Source: three-view drawing plus pictorial views. Frame: mm from the lowest corner of the part. A direction names the side the tool comes from. Round coordinates to 2 decimals unless told otherwise and drop trailing zeros. Write each loop counter-clockwise with the first axis right and the second up, starting at its lowest first coordinate (ties: lowest second). Pieces come first, ordered by that corner, then holes.
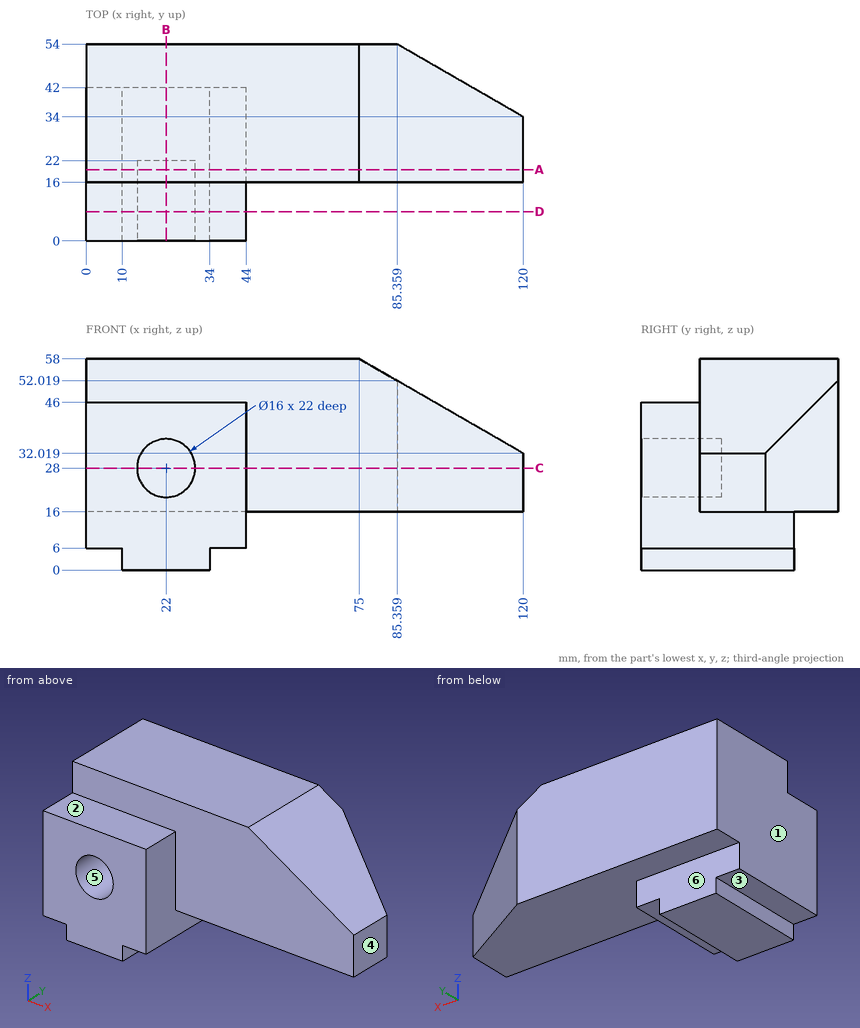
1) Section B-B on x = 22. Output: boundary loops of the cut face in (y, z), plus the area to 3 significant figures.
2) Section D-D on y = 8. Output: boundary loops of the cut face in (x, z).
3) Reachability of the marked faces 1, 2 and 3 from +Z, -Z, +X, -X, +Y, -Y: full face, straight path, thin tool, end or side. Return the list, or none.
4) Section A-A on y = 19.5. Output: boundary loops of the cut face in (x, z).
5) Line query: probe 1 along Z at (x, y) = (22, 5.75); probe 2 along X at (y, z) = (38, 5); probe 3 along Y at (x, z) = (67, 29). Output: solid intervals per line, ascending.
6) Section C-C on z = 28. Output: boundary loops of the cut face in (x, y), plus the area to 3 significant figures.
7) Draft query along X for the marked faces 4, 5 and 6. Return one class per face: pulls with the +X half, pulls with the -X half, needs draft (parallel to the pull), parting line crosses it, or undercut.
8) First-contact query: P1, Ø8, axis at x = 23.5, z = 25, coming from the -Y side; P2, Ø5, axis at y = 19.5, z = 3, coming from the -X side; P3, Ø4, axis at y = 43.5, z = 30.5, coming from the +X side. Flat tips, straight axial feed; report the tip coordinate or a pass-through.
Filled in:
1. outline: (0, 0) - (42, 0) - (42, 16) - (54, 16) - (54, 58) - (16, 58) - (16, 46) - (0, 46) - (0, 36) - (22, 36) - (22, 20) - (0, 20) - close
1. area: 2,400 mm2
2. outline: (0, 6) - (10, 6) - (10, 0) - (34, 0) - (34, 6) - (44, 6) - (44, 46) - (0, 46) - close; hole circle Ø16 at (22, 28)
3. face 1: +Z, -Z, -X, +Y, -Y
3. face 2: +Z, +X, -X, -Y
3. face 3: -Z, -X, +Y, -Y
4. outline: (0, 6) - (10, 6) - (10, 0) - (34, 0) - (34, 6) - (44, 6) - (44, 16) - (120, 16) - (120, 32.02) - (75, 58) - (0, 58) - close; hole circle Ø16 at (22, 28)
5. probe 1: z = 0 to 20, 36 to 46
5. probe 2: x = 10 to 34
5. probe 3: y = 16 to 54
6. outline: (0, 0) - (14, 0) - (14, 22) - (30, 22) - (30, 0) - (44, 0) - (44, 16) - (120, 16) - (120, 34) - (85.36, 54) - (0, 54) - close
6. area: 4,570 mm2
7. face 4: pulls with the +X half
7. face 5: undercut
7. face 6: needs draft
8. P1: stops at y = 22
8. P2: stops at x = 10
8. P3: stops at x = 107.01
